For this review, use the dimensioned drawing (mm, ordinates from the lowest corner) and the shaded views. Give positions to 0.01 mm unless a question says otherwise; leave off trailing zeros. Write each loop counter-clockwise with the first axis right and the second up, starting at its lowest first coordinate (ties: lowest second). Pieces come first, ordered by that corner, then holes. Notation, with made-up numbers: M 27,12.25 L 81,12.25 A33 cw 81,47.25 Z; hole C 62,-20.5 d3. An arc over 180 degrees is marked long. One line per item, written item: value. Start each with the question number.
Item 1: Consider section A-A, the plane z = 88.9. Write out the cut boundary in (x, y) (1 decimal).
Item 2: To check wall thickness, follow probe 1 along X at (y, z) = (2.5, 88.9); probe 2 along Z at (x, y) = (176, 3.25); probe 3 along Z at (x, y) = (170.5, 4) (1 decimal). State the ranges of each line that lie inside material, in increasing order.
Item 3: Clearance check with flat-ended pins moving along their axes: pin 1 Ø4 at (x, y) = (105, 6) entering from -Z; pin 2 Ø6.5 at (x, z) = (50.8, 88.9) entering from -Y. State where each tip first meets the part, or that it passes through.
Item 4: Consider section B-B, the plane x = 50.8. Write out the cut boundary in (y, z) (1 decimal), and give its area (3 significant figures).
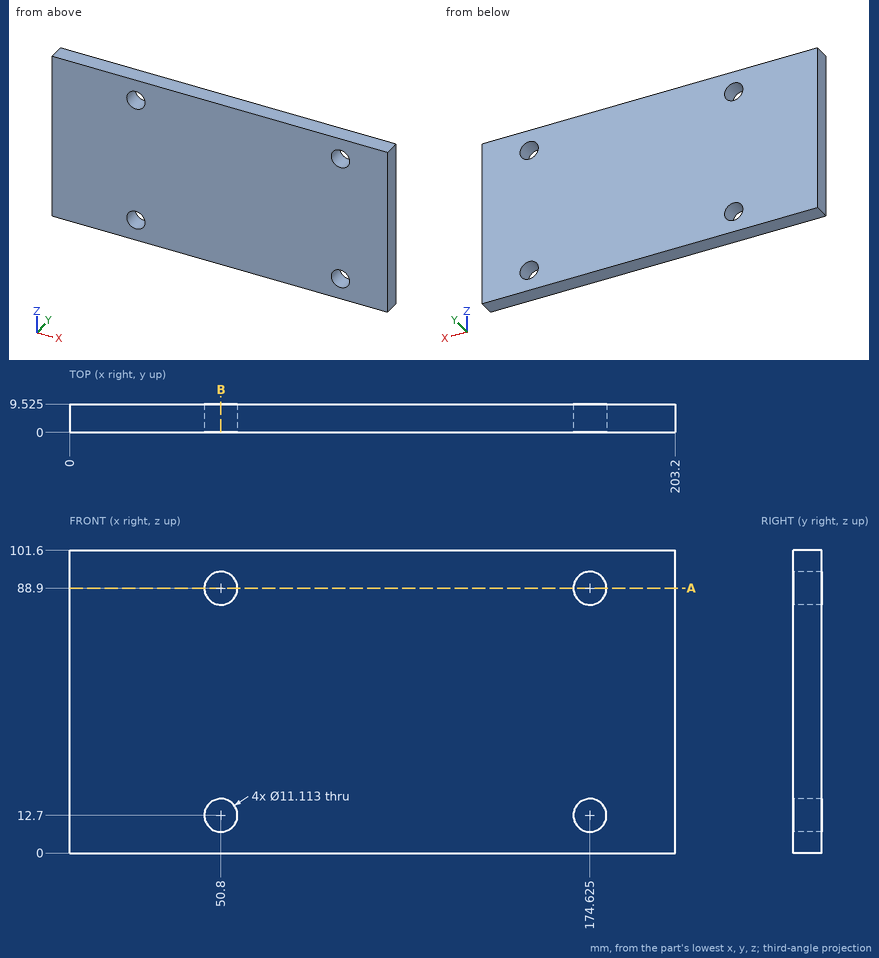
Model answer:
1. outline: M 0,0 L 45.2,0 L 45.2,9.5 L 0,9.5 Z; M 56.4,0 L 169.1,0 L 169.1,9.5 L 56.4,9.5 Z; M 180.2,0 L 203.2,0 L 203.2,9.5 L 180.2,9.5 Z
2. probe 1: x = 0 to 45.24, 56.36 to 169.07, 180.18 to 203.2
2. probe 2: z = 0 to 7.32, 18.08 to 83.52, 94.28 to 101.6
2. probe 3: z = 0 to 9, 16.4 to 85.2, 92.6 to 101.6
3. pin 1: stops at z = 0
3. pin 2: passes through
4. outline: M 0,0 L 9.5,0 L 9.5,7.1 L 0,7.1 Z; M 0,18.3 L 9.5,18.3 L 9.5,83.3 L 0,83.3 Z; M 0,94.5 L 9.5,94.5 L 9.5,101.6 L 0,101.6 Z
4. area: 756 mm2
